Build history of the part. All positions in model axes, mm. Face numbers are marked on the shaded views. A direction names the side the tool comes from. Round coordinates to 2 decimals unless told otherwise and drop trailing zeros. Order: outer loops, then holes, each group sorted by start corner. A loop starts at its lowest first (then second) coordinate and runs counter-clockwise, first axis right, second up. Notation, with made-up numbers: M 17.5,11.25 L 56.5,11.25 A22 cw 56.5,37.25 Z; hole C -34,-16 d11. An arc over 180 degrees is marked long. Use CSV: the item, a comma, the result in double quotes.
from build123d import *

# Parameters (mm, degrees)
SKETCH1_R           = 12.5
SKETCH1_R_2         = 1.6
SKETCH1_R_3         = 1
BOSS_EXTRUDE1_DEPTH = 5
CUT_EXTRUDE1_DEPTH  = 6
CIRPATTERN1_COUNT   = 22


with BuildPart() as part:
    # Sketch1 → Boss-Extrude1 (new body)
    with BuildSketch(Plane.XY):
        Circle(SKETCH1_R)
        Circle(SKETCH1_R_2, mode=Mode.SUBTRACT)
        with Locations((-2.5, 7.4)):
            Circle(SKETCH1_R_3, mode=Mode.SUBTRACT)
        with Locations((2.5, 7.4)):
            Circle(SKETCH1_R_3, mode=Mode.SUBTRACT)
        with Locations((2.5, -7.4)):
            Circle(SKETCH1_R_3, mode=Mode.SUBTRACT)
        with Locations((-2.5, -7.4)):
            Circle(SKETCH1_R_3, mode=Mode.SUBTRACT)
        with Locations((7.4, -2.5)):
            Circle(SKETCH1_R_3, mode=Mode.SUBTRACT)
        with Locations((7.4, 2.5)):
            Circle(SKETCH1_R_3, mode=Mode.SUBTRACT)
        with Locations((-7.4, 2.5)):
            Circle(SKETCH1_R_3, mode=Mode.SUBTRACT)
        with Locations((-7.4, -2.5)):
            Circle(SKETCH1_R_3, mode=Mode.SUBTRACT)
    extrude(amount=BOSS_EXTRUDE1_DEPTH)

    # Sketch2 → Cut-Extrude1 (cut, through all)
    with BuildSketch(Plane.XY.offset(5)):
        Polygon((-5.188791036, 11.579242099), (-7.447104706, 10.054235749), (-5.067298356, 8.22762092), (-4.383588712, 8.68932009), align=None)
    cut_extrude1 = extrude(amount=-CUT_EXTRUDE1_DEPTH, mode=Mode.SUBTRACT)

    # CirPattern1: Cut-Extrude1 ×22 about axis
    cirpattern1_axis = Axis((0, 0, 0), (0, 0, 1))
    for i in range(1, CIRPATTERN1_COUNT):
        add(cut_extrude1.rotate(cirpattern1_axis, i * 360 / CIRPATTERN1_COUNT), mode=Mode.SUBTRACT)


solid = part.part
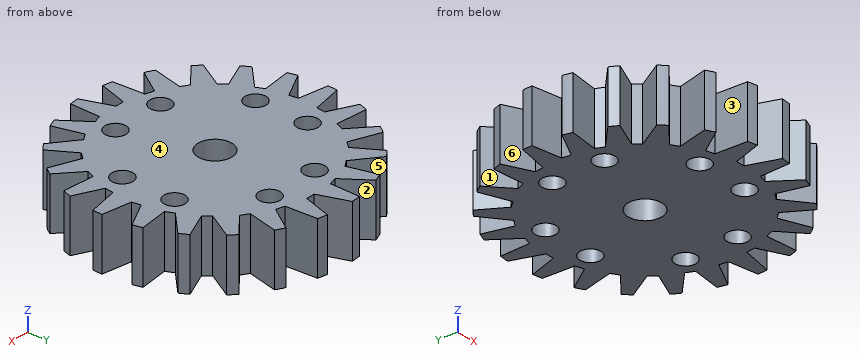
(1) Tool access for the marked faces 1, 2 and 3: list every direction of +Z, -Z, +X, -X, +Y, -Y with a clear straight run to the whole face (end or side of a thin tool).
Answer block:
face 1,"+Z, -Z, -X"
face 2,"+Z, -Z, +Y"
face 3,"+Z, -Z, -Y"
(2) Cut at B-B, the plane z = 1.85. Count the separate pieces of the cut face and the enclosed holes in it, and give its area (3 significant figures).
Answer block:
separate pieces,"1"
enclosed holes,"9"
area,"350 mm²"
(3) Cut at A-A, the plane x = 2.25. Give the cut face in (y, z).
Answer block:
outline,"M -9.42,0 L -8.37,0 L -8.37,5 L -9.42,5 Z; M -6.43,0 L 6.43,0 L 6.43,5 L -6.43,5 Z; M 8.37,0 L 12.3,0 L 12.3,5 L 8.37,5 Z"
(4) Two-plate mould, pull along X, no slides. Class the marked faces 4, 5 and 6: released by +X, released by -X, zero draft, split by the parting line, or undercut.
Answer block:
face 4,"zero draft"
face 5,"undercut"
face 6,"released by -X"
(5) Drop flat-ended pins along their axis: pin 1 (1.8 mm diameter, centred on x = -2.5, y = 7.4, fed in from +Z); pin 2 (2 mm diameter, centred on y = -3.5, z = 1.5, fed in from +X). Give the stop position or say it passes through.
Answer block:
pin 1,"passes through"
pin 2,"stops at x = 11.98"
(6) Wall check: line 1 (Y direction, x = -2.5, z = 1.1); line 2 (Y direction, x = -8, z = 1.65); line 3 (X direction, y = 8.75, z = 3.45). Give the ranges that are in metal, low to high. Write a range as from..to.
Answer block:
line 1,"y = -12.25..-8.4, -6.4..6.4, 8.4..9.34"
line 2,"y = -9.21..-7.21, -5.59..-3.3, -1.7..1.7, 3.3..6.78, 9.26..9.6"
line 3,"x = -7.68..-5.75, -4.4..5.55, 7.45..8.86"
